Verification items for the finished model (mm, model axes). Face numbers are marked on the shaded views. A direction names the side the tool comes from. Round coordinates to 2 decimals unless told otherwise and drop trailing zeros. Loops run counter-clockwise (first coordinate to the right, second up) from the corner with the lowest first, then second, coordinate; pieces in that order, holes last. Notation, with made-up numbers: M 63.5,46.25 L 121.5,46.25 A31 cw 121.5,71.25 Z; hole C 2,-9.75 d11. An arc over 180 degrees is marked long. Answer as CSV lines item,"result".
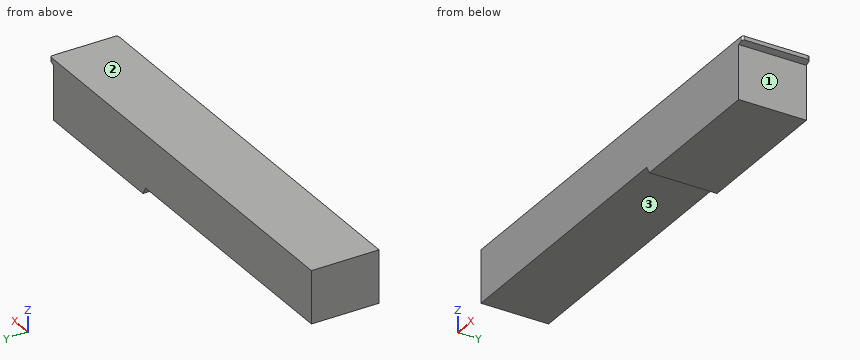
```python
from build123d import *

# Parameters (mm, degrees)
SKETCH1_W               = 22.5
SKETCH1_H               = 142
BOSS_EXTRUDE1_DEPTH     = 20
SKETCH2_W               = 22.5
SKETCH2_H               = 18
CUT_EXTRUDE1_DEPTH      = 2
CHAMFER5_SIZE           = 2.060608065
CHAMFER5_SIZE_2         = 0.75
FILLET5_R               = 0.75
CUT_EXTRUDE4_DEPTH      = 146.155950619
CUT_EXTRUDE4_DEPTH_BACK = 146.155950619


with BuildPart() as part:
    # Sketch1 → Boss-Extrude1 (new body)
    with BuildSketch(Plane(origin=(0, 0, 0), x_dir=(0, 1, 0), z_dir=(0, 0, 1))):
        with Locations((11.25, -71)):
            Rectangle(SKETCH1_W, SKETCH1_H)
    extrude(amount=-BOSS_EXTRUDE1_DEPTH)

    # Sketch2 → Cut-Extrude1 (cut)
    with BuildSketch(Plane.YZ.offset(142)):
        with Locations((11.25, -11)):
            Rectangle(SKETCH2_W, SKETCH2_H)
    extrude(amount=-CUT_EXTRUDE1_DEPTH, mode=Mode.SUBTRACT)

    # Chamfer5
    # the kernel refuses this chamfer: 2.060608065, 0.75 mm, written as the material it takes off along each edge
    with BuildSketch(Plane(origin=(142, 27.845618587, -2), x_dir=(-0.9999130865277316, 0, -0.013184058198645886), z_dir=(0, -1, 0))) as chamfer5_piece_1_section:
        Polygon((CHAMFER5_SIZE * 0.999913086329, -CHAMFER5_SIZE * 0.013184058196), (-CHAMFER5_SIZE_2 * 0.0131840581986, -CHAMFER5_SIZE_2 * 0.999913086528), (0, 0), align=None)
    chamfer5_piece_1 = extrude(amount=33.191237174, mode=Mode.PRIVATE)
    chamfer5_piece_1 = split(chamfer5_piece_1, bisect_by=Plane(origin=(140, 11.25, -1.766801206), z_dir=(1, 0, 0)), keep=Keep.TOP, mode=Mode.PRIVATE)
    add(chamfer5_piece_1, mode=Mode.SUBTRACT)

    # Fillet5
    fillet5_edges = [part.edges().sort_by_distance(p)[0] for p in [
        (142, 0, -0.625),
        (142, 22.5, -0.625),
    ]]
    fillet(fillet5_edges, radius=FILLET5_R)

    # Sketch6 → Cut-Extrude4 (cut, two sides: drawn at the far end of the back side and taken through both)
    with BuildSketch(Plane(origin=(0, 22.5, 0), x_dir=(-1, 0, 0), z_dir=(0, 1, 0)).offset(-CUT_EXTRUDE4_DEPTH_BACK)):
        Polygon((0, -17.5), (-90, -17.5), (-91.5, -20), (-90, -20), (0, -20), align=None)
    extrude(amount=CUT_EXTRUDE4_DEPTH + CUT_EXTRUDE4_DEPTH_BACK, mode=Mode.SUBTRACT)


solid = part.part
```
1) Set-up check for the marked faces 1, 2 and 3: record each of +Z, -Z, +X, -X, +Y, -Y from which the full face is reachable in a straight line by a thin tool's end or side.
Here are the results:
face 1,"-Z, +X, +Y, -Y"
face 2,"+Z, +X, -X, +Y, -Y"
face 3,"-Z, -X, +Y, -Y"
2) Section check A-A (y = 19.25). Record the cut outline in (x, z), plus the area to 3 significant figures.
Here are the results:
outline,"M 0,-17.5 L 90,-17.5 L 91.5,-20 L 140,-20 L 140,-1.98 L 142,-1.25 L 142,0 L 0,0 Z"
area,"2,580 mm^2"
3) Go/stop test with flat-tipped pins: pin 1 (9 mm diameter, centred on y = 12.5, z = -10.5, fed in from +X); pin 2 (11 mm diameter, centred on x = 44, y = 16.5, fed in from -Z). Record where each tip stops, or that it passes through.
Here are the results:
pin 1,"stops at x = 140"
pin 2,"stops at z = -17.5"
4) Material ranges on probe 1 along X at (y, z) = (19.75, -5.75); probe 2 along Z at (x, y) = (50, 20.75); probe 3 along X at (y, z) = (6.25, -18.75), recorded low to high.
Here are the results:
probe 1,"x = 0 to 140"
probe 2,"z = -17.5 to 0"
probe 3,"x = 90.75 to 140"
5) Section check B-B (x = 27.5). Record the cut outline in (y, z).
Here are the results:
outline,"M 0,-17.5 L 22.5,-17.5 L 22.5,0 L 0,0 Z"
